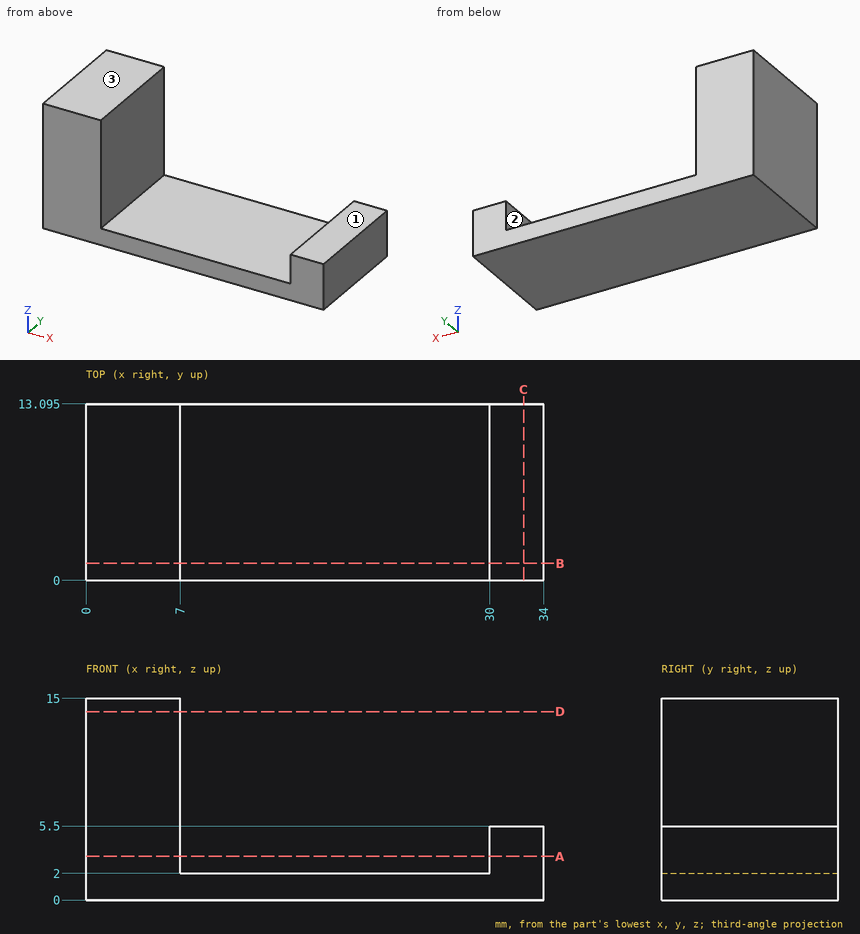
Geometry: see drawing. Coordinates: mm, zero at the bounding-box minimum. A direction names the side the tool comes from. Give positions to 0.01 mm unless a question says otherwise; leave off trailing zeros. Order: outer loops, then holes, each group sorted by start corner. A loop starts at its lowest first (then second) coordinate and runs counter-clockwise, first axis right, second up. Notation, with made-up numbers: (69.25, 32.25) - (104.25, 32.25) arc R16 cw to (104.25, 46.25) - close; hole circle Ø7 at (54.5, 64). An arc over 180 degrees is marked (long way). Write each question's results on one line, items separated by ' | '.
Item 1: Section B-B (y = 1.25). Return loops of the section in (x, z).
A:
outline: (0, 0) - (34, 0) - (34, 5.5) - (30, 5.5) - (30, 2) - (7, 2) - (7, 15) - (0, 15) - close
Item 2: Contact query for flat-ended pins moving along their axis: pin 1 Ø6 at (x, y) = (25, 1.5) entering from +Z; pin 2 Ø2 at (x, y) = (32, 5) entering from +Z; pin 3 Ø2 at (y, z) = (6, 7.5) entering from +X. Output: stop coordinate, or through.
A:
pin 1: stops at z = 2 | pin 2: stops at z = 5.5 | pin 3: stops at x = 7
Item 3: Access query for the marked faces 1, 2 and 3. Directions: +Z, -Z, +X, -X, +Y, -Y. A direction counts if a zero-diameter tool reaches every point of the face in a straight line with its end or side. Return the directions, or none.
A:
face 1: +Z, +X, +Y, -Y | face 2: +Z, +Y, -Y | face 3: +Z, +X, -X, +Y, -Y
Item 4: Section D-D (z = 14). Return loops of the section in (x, y) (1 decimal).
A:
outline: (0, 0) - (7, 0) - (7, 13.1) - (0, 13.1) - close
Item 5: Section A-A (z = 3.25). Return loops of the section in (x, y) (1 decimal), and give its area (3 significant figures).
A:
outline: (0, 0) - (7, 0) - (7, 13.1) - (0, 13.1) - close; (30, 0) - (34, 0) - (34, 13.1) - (30, 13.1) - close | area: 144 mm^2
Item 6: Material intervals for line 1 along X through (y, z) = (12, 2.5); line 2 along Z through (x, y) = (17.5, 8.75); line 3 along Z through (x, y) = (32, 9.25), sorted ascending.
A:
line 1: x = 0 to 7, 30 to 34 | line 2: z = 0 to 2 | line 3: z = 0 to 5.5
Item 7: Section C-C (x = 32.5). Return loops of the section in (y, z) (1 decimal), and give its area (3 significant figures).
A:
outline: (0, 0) - (13.1, 0) - (13.1, 5.5) - (0, 5.5) - close | area: 72.0 mm^2
